Check sheet for the modelled part. Datum: model origin and axes. Units: mm. A direction names the side the tool comes from. Coordinates: 2 decimals unless noted, no trailing zeros. Loops run counter-clockwise (first coordinate to the right, second up) from the corner with the lowest first, then second, coordinate; pieces in that order, holes last.
from build123d import *

# Parameters (mm, degrees)
SKETCH1_R           = 38.1
SKETCH1_R_2         = 22.225
BOSS_EXTRUDE1_DEPTH = 12.7
SKETCH2_W           = 101.6
SKETCH2_H           = 25.4
BOSS_EXTRUDE2_DEPTH = 38.1
SKETCH3_R           = 12.7
CUT_EXTRUDE1_DEPTH  = 195.272643468
SKETCH4_R           = 9.525
CUT_EXTRUDE3_DEPTH  = 38.1
FILLET3_R           = 25.4
SKETCH6_W           = 101.6
SKETCH6_H           = 25.4
BOSS_EXTRUDE3_DEPTH = 38.1
SKETCH7_R           = 12.7
CUT_EXTRUDE4_DEPTH  = 195.272643468
SKETCH8_R           = 9.525
CUT_EXTRUDE5_DEPTH  = 195.272643468
FILLET4_R           = 25.4


with BuildPart() as part:
    # Sketch1 → Boss-Extrude1 (new, symmetric)
    # profile 1 of 2: a face of its own
    with BuildSketch(Plane(origin=(0, 0, 0), x_dir=(1, 0, 0), z_dir=(0, 1, 0))):
        with BuildLine():
            Line((0, 25.4), (0, 0))
            Line((0, 0), (127, 0))
            Line((127, 0), (159.995567884, 57.15))
            ThreePointArc((159.995567884, 57.15), (101.997796947, 47.451089716), (103.55657019, 106.233574525))
            Line((103.55657019, 106.233574525), (0, 25.4))
        make_face()
    # profile 2 of 2: a face of its own
    with BuildSketch(Plane(origin=(0, 0, 0), x_dir=(1, 0, 0), z_dir=(0, 1, 0))):
        with Locations((127, 76.2)):
            Circle(SKETCH1_R)
        with Locations(Location((127, 76.2, 0), (0, 0, 270))):
            Circle(SKETCH1_R_2, mode=Mode.SUBTRACT)
    extrude(amount=BOSS_EXTRUDE1_DEPTH, both=True)

    # Sketch2 → Boss-Extrude2 (add)
    with BuildSketch(Plane(origin=(0, 12.7, 0), x_dir=(1, 0, 0), z_dir=(0, 1, 0))):
        with Locations((50.8, 12.7)):
            Rectangle(SKETCH2_W, SKETCH2_H)
    extrude(amount=BOSS_EXTRUDE2_DEPTH)

    # Sketch3 → Cut-Extrude1 (cut, through all)
    with BuildSketch(Plane(origin=(0, 0, -25.4), x_dir=(-1, 0, 0), z_dir=(0, 0, -1))):
        with BuildLine():
            ThreePointArc((-101.6, 25.4), (-88.9, 38.1), (-76.2, 25.4))
            Line((-76.2, 25.4), (-76.2, 50.8))
            Line((-76.2, 50.8), (-101.6, 50.8))
            Line((-101.6, 50.8), (-101.6, 25.4))
        make_face()
        with Locations((-88.9, 25.4)):
            Circle(SKETCH3_R)
        with BuildLine():
            Line((-101.6, 12.7), (-88.9, 12.7))
            ThreePointArc((-88.9, 12.7), (-97.880256121, 16.419743879), (-101.6, 25.4))
            Line((-101.6, 25.4), (-101.6, 12.7))
        make_face()
    extrude(amount=-CUT_EXTRUDE1_DEPTH, mode=Mode.SUBTRACT)

    # Sketch4 → Cut-Extrude3 (cut)
    with BuildSketch(Plane(origin=(0, 0, -25.4), x_dir=(-1, 0, 0), z_dir=(0, 0, -1))):
        with Locations((-38.1, 31.75)):
            Circle(SKETCH4_R)
    extrude(amount=-CUT_EXTRUDE3_DEPTH, mode=Mode.SUBTRACT)

    # Fillet3
    fillet3_edges = [part.edges().sort_by_distance(p)[0] for p in [
        (0, 50.8, -12.7),
    ]]
    fillet(fillet3_edges, radius=FILLET3_R)

    # Sketch6 → Boss-Extrude3 (add)
    with BuildSketch(Plane.XZ.offset(12.7)):
        with Locations((50.8, -12.7)):
            Rectangle(SKETCH6_W, SKETCH6_H)
    extrude(amount=BOSS_EXTRUDE3_DEPTH)

    # Sketch7 → Cut-Extrude4 (cut, through all)
    with BuildSketch(Plane(origin=(0, 0, -25.4), x_dir=(-1, 0, 0), z_dir=(0, 0, -1))):
        with BuildLine():
            Line((-76.2, -50.8), (-76.2, -25.4))
            ThreePointArc((-76.2, -25.4), (-88.9, -38.1), (-101.6, -25.4))
            Line((-101.6, -25.4), (-101.6, -50.8))
            Line((-101.6, -50.8), (-76.2, -50.8))
        make_face()
        with Locations((-88.9, -25.4)):
            Circle(SKETCH7_R)
        with BuildLine():
            ThreePointArc((-101.6, -25.4), (-97.880256121, -16.419743879), (-88.9, -12.7))
            Line((-88.9, -12.7), (-101.6, -12.7))
            Line((-101.6, -12.7), (-101.6, -25.4))
        make_face()
    extrude(amount=-CUT_EXTRUDE4_DEPTH, mode=Mode.SUBTRACT)

    # Sketch8 → Cut-Extrude5 (cut, through all)
    with BuildSketch(Plane(origin=(0, 0, -25.4), x_dir=(-1, 0, 0), z_dir=(0, 0, -1))):
        with Locations((-38.1, -31.75)):
            Circle(SKETCH8_R)
    extrude(amount=-CUT_EXTRUDE5_DEPTH, mode=Mode.SUBTRACT)

    # Fillet4
    fillet4_edges = [part.edges().sort_by_distance(p)[0] for p in [
        (0, -50.8, -12.7),
    ]]
    fillet(fillet4_edges, radius=FILLET4_R)


solid = part.part
(1) Draft check along X on faces 5 (the face through (100, 12.7, -58)), 6 (the face through (80.02, 16.32, -12.88)), 7 (the face through (33.7, -40.2, -12.9)), 8 (the face through (7.24, -43.16, -12.52)). Enter one of: pulls with the +X half, pulls with the -X half, needs draft (parallel to the pull), parting line crosses it, or undercut.
(2) Section check D-D, the plane y = 10. Enter the section's corners in (x, z) (3 decimals).
(3) Section check B-B, the plane z = -76. Enter the section's corners in (x, y), plus the area to 3 significant figures.
(4) Scan lines: line 1 along Y through (x, z) = (38, -15); line 2 along Y through (x, z) = (31.5, -20); line 3 along Y through (x, z) = (101.5, -78). Record each from-to range of solid material in increasing order.
(5) Set-up check for faces 1 (the face through (100, -12.7, -58)), 2 (the face through (76.2, -38, -13)), 3 (the face through (76.2, 38, -13)), 4 (the face through (33.7, 23.3, -12.9)): record each of +Z, -Z, +X, -X, +Y, -Y from which the full face is reachable in a straight line by a thin tool's end or side.
(6) Section check C-C, the plane x = 34.5. Enter the section's corners in (y, z), plus the area to 3 significant figures.
(7) Section check A-A, the plane x = 130. Enter the section's corners in (y, z).
(8) Gauge pin test, flat ends, axial feed: P1, Ø8, axis at y = 2.5, z = -41, coming from the +X side; P2, Ø1.5, axis at y = 12.5, z = -99, coming from the +X side; P3, Ø12.5, axis at y = -37.5, z = -18.5, coming from the +X side. Record the tip position at first contact, or that the pin passes through.
Determined:
1. face 5: needs draft
1. face 6: pulls with the +X half
1. face 7: undercut
1. face 8: pulls with the -X half
2. outline: (0, -25.4) - (103.557, -106.234) arc R38.1 ccw to (159.996, -57.15) - (127, 0) - (0, 0) - close; hole circle Ø44.45 at (127, -76.2)
3. outline: (64.82, -12.7) - (104.78, -12.7) - (104.78, 12.7) - (64.82, 12.7) - close; (149.22, -12.7) - (165.1, -12.7) - (165.1, 12.7) - (149.22, 12.7) - close
3. area: 1,420 mm2
4. line 1: y = -50.8 to -41.27, -22.23 to 22.23, 41.27 to 50.8
4. line 2: y = -50.8 to -38.62, -24.88 to 24.88, 38.62 to 50.8
4. line 3: y = -12.7 to 12.7
5. face 1: -Z, +X, -Y
5. face 2: +Z, -Z, +X, -Y
5. face 3: +Z, -Z, +X, +Y
5. face 4: +Z, -Z
6. outline: (-50.8, -25.4) - (-40.57, -25.4) - (-40.57, 0) - (-50.8, 0) - close; (-22.93, -25.4) - (-12.7, -25.4) - (-12.7, -52.33) - (12.7, -52.33) - (12.7, -25.4) - (22.93, -25.4) - (22.93, 0) - (-22.93, 0) - close; (40.57, -25.4) - (50.8, -25.4) - (50.8, 0) - (40.57, 0) - close
6. area: 2,370 mm2
7. outline: (-12.7, -114.18) - (12.7, -114.18) - (12.7, -98.22) - (-12.7, -98.22) - close; (-12.7, -54.18) - (12.7, -54.18) - (12.7, -5.2) - (-12.7, -5.2) - close
8. P1: stops at x = 152.98
8. P2: stops at x = 158.07
8. P3: stops at x = 76.2
